Source: CAD feature listing. Evaluate the final solid. Frame: model axes, mm. A direction names the side the tool comes from. Coordinates: 2 decimals unless noted, no trailing zeros. Loops run counter-clockwise (first coordinate to the right, second up) from the corner with the lowest first, then second, coordinate; pieces in that order, holes last. Notation, with made-up numbers: M -38.75,-2 L 12.25,-2 A22 cw 12.25,36 Z; hole C 65.5,6 d4. An arc over 180 degrees is marked long. One line per question, with ' | ' between items. Start each with the question number.
1. Section query A-A, the plane x = 51. Output: boundary loops of the cut face in (y, z), and give its area (3 significant figures).
2. Mould query, pull axis Y, two halves, no side actions, for faces 1 (the flat face through (-40, -33.951, 34)), 2 (the flat face through (29, -40, 38.329)), 3 (the flat face through (52, 4.44, 7)), 4 (the flat face through (14, 25.504, 15)). Classes: pulls with the +Y half, pulls with the -Y half, needs draft (parallel to the pull), parting line crosses it, or undercut.
3. Ray query, probe 1 along X at (y, z) = (4.5, 28); probe 2 along Y at (x, z) = (-46.5, 34); probe 3 along X at (y, z) = (3, 9). Return the intervals inside material, ascending.
4. Access query for faces 5 (the flat face through (29, 13.231, 34)), 6 (the flat face through (-47.519, -9, 24)), 7 (the flat face through (37.317, -10, 24)). Directions: +Z, -Z, +X, -X, +Y, -Y. A direction counts if a zero-diameter tool reaches every point of the face in a straight line with its end or side. Return the directions, or none.
5. Section query B-B, the plane y = -31. Output: boundary loops of the cut face in (x, z).
6. Section query D-D, the plane z = 16. Output: boundary loops of the cut face in (x, y), and give its area (3 significant figures).
7. Pin query (flat end, axial travel): P1, Ø11.5, axis at y = -10, z = 5, coming from the +X side; P2, Ø10, axis at x = 24, z = 22, coming from the +Y side; P3, Ø3, axis at x = 42, y = 5.5, coming from the +Z side. Return the tip coordinate at first contact, or that it passes through.
8. Section query C-C, the plane x = -39. Output: boundary loops of the cut face in (y, z).
```python
from build123d import *

# Parameters (mm, degrees)
F0_W      = 53.3400028944
F0_H      = 70.8285234869
F1_DEPTH  = 25.4
F2_R      = 8.4728642263
F3_DEPTH  = 41.402
F4_W      = 70.9742624313
F4_H      = 38.3290164173
F5_DEPTH  = 15.748
F6_W      = 70.9742605686
F6_H      = 38.3290164173
F7_DEPTH  = 15.748
F8_W      = 70.9742624313
F8_H      = 14.1365574673
F9_DEPTH  = 23.114
F10_W     = 70.9742605686
F10_H     = 14.3422139809
F11_DEPTH = 23.114
F12_W     = 16.9909100647
F12_H     = 25.4818284884
F13_DEPTH = 25.4
F14_W     = 15.8581200655
F14_H     = 25.6498372182
F15_DEPTH = 25.4
F16_W     = 47.4318256602
F16_H     = 7.9976115376
F17_DEPTH = 25.4
F18_W     = 47.4318237975
F18_H     = 7.9976115376
F19_DEPTH = 25.4


with BuildPart() as f1:
    # F0 (on Top) → F1 (new body)
    with BuildSketch(Plane.XY):
        with Locations((-5.1008202136, -9.9101644009)):
            Rectangle(F0_W, F0_H)
    extrude(amount=F1_DEPTH)

    # F2 (on face) → F3 (cut)
    with BuildSketch(Plane.XY.offset(25.4)):
        with Locations((-4.66360664, -7.4326233007)):
            Circle(F2_R)
    extrude(amount=-F3_DEPTH, mode=Mode.SUBTRACT)

    # F4 (on face) → F5 (join)
    with BuildSketch(Plane(origin=(-31.7708216608, 0, 0), x_dir=(0, -1, 0), z_dir=(-1, 0, 0))):
        with Locations((9.8372949287, 19.1645082086)):
            Rectangle(F4_W, F4_H)
    extrude(amount=F5_DEPTH)

    # F6 (on face) → F7 (join)
    with BuildSketch(Plane.YZ.offset(21.5691812336)):
        with Locations((-9.9830329418, 19.1645082086)):
            Rectangle(F6_W, F6_H)
    extrude(amount=F7_DEPTH)

    # F8 (on face) → F9 (join)
    with BuildSketch(Plane(origin=(-47.5188216608, 0, 0), x_dir=(0, -1, 0), z_dir=(-1, 0, 0))):
        with Locations((9.8372949287, 7.0682787336)):
            Rectangle(F8_W, F8_H)
    extrude(amount=F9_DEPTH)

    # F10 (on face) → F11 (join)
    with BuildSketch(Plane.YZ.offset(37.3171812336)):
        with Locations((-9.9830329418, 7.1711069904)):
            Rectangle(F10_W, F10_H)
    extrude(amount=F11_DEPTH)

    # F12 (on face) → F13 (cut)
    with BuildSketch(Plane.XY.offset(14.3422139809)):
        with Locations((51.9357262013, -8.3012259565)):
            Rectangle(F12_W, F12_H)
    extrude(amount=-F13_DEPTH, mode=Mode.SUBTRACT)

    # F14 (on face) → F15 (cut)
    with BuildSketch(Plane.XY.offset(14.1365574673)):
        with Locations((-62.703761628, -8.7442626245)):
            Rectangle(F14_W, F14_H)
    extrude(amount=-F15_DEPTH, mode=Mode.SUBTRACT)

    # F16 (on face) → F17 (cut)
    with BuildSketch(Plane(origin=(21.5691812336, 0, 0), x_dir=(0, -1, 0), z_dir=(-1, 0, 0))):
        with Locations((10.4849305935, 34.3302106485)):
            Rectangle(F16_W, F16_H)
    extrude(amount=-F17_DEPTH, mode=Mode.SUBTRACT)

    # F18 (on face) → F19 (cut)
    with BuildSketch(Plane.YZ.offset(-31.7708216608)):
        with Locations((-10.2352886461, 34.3302106485)):
            Rectangle(F18_W, F18_H)
    extrude(amount=-F19_DEPTH, mode=Mode.SUBTRACT)


solid = f1.part
```
Taken from the geometry:
1) outline: M -45.47,0 L -21.04,0 L -21.04,14.34 L -45.47,14.34 Z; M 4.44,0 L 25.5,0 L 25.5,14.34 L 4.44,14.34 Z | area: 652 mm^2
2) face 1: undercut | face 2: needs draft | face 3: undercut | face 4: pulls with the +Y half
3) probe 1: -47.52 to -31.77, 21.57 to 37.32 | probe 2: -45.32 to -33.95, 13.48 to 25.65 | probe 3: -54.77 to 43.44
4) face 5: +Z, +X, -X | face 6: +Z, -X, +Y, -Y | face 7: +Z, +X, +Y, -Y
5) outline: M -70.63,0 L 60.43,0 L 60.43,14.34 L 37.32,14.34 L 37.32,30.33 L 21.57,30.33 L 21.57,25.4 L -31.77,25.4 L -31.77,30.33 L -47.52,30.33 L -47.52,14.14 L -70.63,14.14 Z
6) outline: M -47.52,-45.32 L 21.57,-45.32 L 21.57,-45.47 L 37.32,-45.47 L 37.32,25.5 L -31.77,25.5 L -31.77,25.65 L -47.52,25.65 Z; hole C -4.66,-7.43 d16.95 | area: 5,790 mm^2
7) P1: x = 43.44 | P2: y = 25.5 | P3: z = 14.34
8) outline: M -45.32,0 L 25.65,0 L 25.65,38.33 L 13.48,38.33 L 13.48,30.33 L -33.95,30.33 L -33.95,38.33 L -45.32,38.33 Z
